Verification items for the finished model (mm, model axes). Face numbers are marked on the shaded views. A direction names the side the tool comes from. Round coordinates to 2 decimals unless told otherwise and drop trailing zeros. Write each loop counter-clockwise with the first axis right and the second up, starting at its lowest first coordinate (ties: lowest second). Pieces come first, ordered by that corner, then holes. Notation, with made-up numbers: M -16.5,53.5 L 13.5,53.5 A12 cw 13.5,74.5 Z; hole C 86,9 d1. An arc over 180 degrees is marked long. Write each question's results on one line, items separated by ' | '.
from build123d import *

# Parameters (mm, degrees)
ESQUISSE2_W             = 44
ESQUISSE2_H             = 44
BOSS_EXTRU_1_DEPTH      = 10
ESQUISSE3_W             = 36
ESQUISSE3_H             = 36
BOSS_EXTRU_2_DEPTH      = 10
ESQUISSE4_W             = 42.5
ESQUISSE4_H             = 42.5
ESQUISSE4_W_2           = 36
ESQUISSE4_H_2           = 36
ENL_V_MAT_EXTRU_1_DEPTH = 5
CONG_1_R                = 3
CONG_2_R                = 2


with BuildPart() as part:
    # Esquisse2 → Boss.-Extru.1 (new body)
    with BuildSketch(Plane.XY):
        with Locations((22, 22)):
            Rectangle(ESQUISSE2_W, ESQUISSE2_H)
    extrude(amount=BOSS_EXTRU_1_DEPTH)

    # Esquisse3 → Boss.-Extru.2 (add)
    with BuildSketch(Plane(origin=(0, 0, 0), x_dir=(-1, 0, 0), z_dir=(0, 0, -1))):
        with Locations((-22, 22)):
            Rectangle(ESQUISSE3_W, ESQUISSE3_H)
    extrude(amount=BOSS_EXTRU_2_DEPTH)

    # Esquisse4 → Enlèv. mat.-Extru.1 (cut)
    with BuildSketch(Plane(origin=(0, 0, 0), x_dir=(-1, 0, 0), z_dir=(0, 0, -1))):
        with Locations((-22.75, 21.25)):
            Rectangle(ESQUISSE4_W, ESQUISSE4_H)
        with Locations((-22, 22)):
            Rectangle(ESQUISSE4_W_2, ESQUISSE4_H_2, mode=Mode.SUBTRACT)
    extrude(amount=-ENL_V_MAT_EXTRU_1_DEPTH, mode=Mode.SUBTRACT)

    # Congé1
    cong_1_edges = [part.edges().sort_by_distance(p)[0] for p in [
        (22, 40, -10),
        (4, 22, -10),
        (22, 4, -10),
        (40, 22, -10),
        (44, 0, 7.5),
        (44, 44, 5),
        (0, 0, 5),
        (0, 44, 5),
        (1.5, 42.5, 2.5),
        (4, 4, -2.5),
        (4, 40, -2.5),
        (40, 4, -2.5),
        (40, 40, -2.5),
    ]]
    fillet(cong_1_edges, radius=CONG_1_R)

    # Congé2
    cong_2_edges = [part.edges().sort_by_distance(p)[0] for p in [
        (44, 22, 10),
        (22, 0, 10),
        (0, 22, 10),
        (22, 44, 10),
        (0.878679656, 43.121320344, 10),
        (0.878679656, 0.878679656, 10),
        (43.121320344, 43.121320344, 10),
        (43.121320344, 0.878679656, 10),
    ]]
    fillet(cong_2_edges, radius=CONG_2_R)


solid = part.part
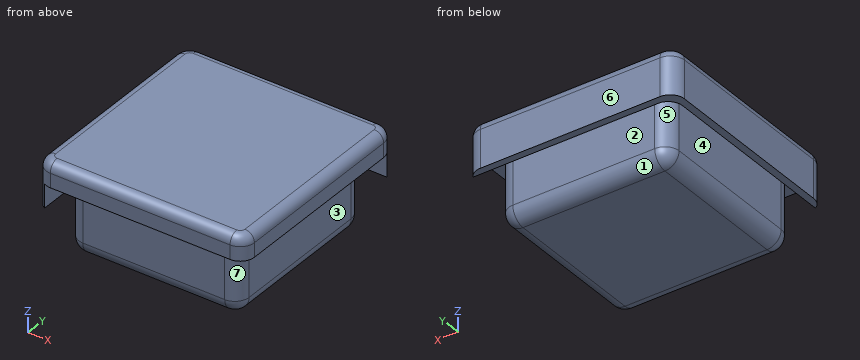
1) Access from +Z, -Z, +X, -X, +Y, -Y to the whole of each face (thin tool, end or side, straight path). Record for the marked faces 1, 2 and 3.
Calculated:
face 1: -Z, +X, -X, +Y | face 2: -Z, +X | face 3: -Z, +X, -Y
2) Depth check by flat-ended pin: P1, Ø3, axis at x = 14, z = 3, coming from the -Y side; P2, Ø5.5, axis at x = 14.5, z = 3, coming from the -Y side; P3, Ø8, axis at y = 20, z = -5, coming from the -X side; P4, Ø3, axis at y = 15.5, z = 1, coming from the +X side. Enter the tip coordinate at first touch or a pass-through.
Calculated:
P1: stops at y = 4 | P2: stops at y = 0 | P3: stops at x = 4 | P4: stops at x = 40
3) Sectioned sample at C-C, the plane z = -5.75. Record the cut outline in (x, y).
Calculated:
outline: M 4,7 A3 ccw 7,4 L 37,4 A3 ccw 40,7 L 40,37 A3 ccw 37,40 L 7,40 A3 ccw 4,37 Z
4) Sectioned sample at A-A, the plane z = 2.75. Record the cut outline in (x, y).
Calculated:
outline: M 0,3 A3 ccw 1.5,0.4 L 1.5,39.5 A3 cw 4.5,42.5 L 43.6,42.5 A3 ccw 41,44 L 3,44 A3 ccw 0,41 Z; M 4,7 A3 ccw 7,4 L 37,4 A3 ccw 40,7 L 40,37 A3 ccw 37,40 L 7,40 A3 ccw 4,37 Z
5) Sectioned sample at B-B, the plane x = 24.5. Record the cut outline in (y, z), and give its area (3 significant figures).
Calculated:
outline: M 0,5 L 4,5 L 4,-7 A3 ccw 7,-10 L 37,-10 A3 ccw 40,-7 L 40,5 L 42.5,5 L 42.5,0 L 44,0 L 44,8 A2 ccw 42,10 L 2,10 A2 ccw 0,8 Z | area: 762 mm²
6) Sectioned sample at D-D, the plane y = 33. Record the cut outline in (x, z), and give its area (3 significant figures).
Calculated:
outline: M 0,0 L 1.5,0 L 1.5,5 L 4,5 L 4,-7 A3 ccw 7,-10 L 37,-10 A3 ccw 40,-7 L 40,5 L 44,5 L 44,8 A2 ccw 42,10 L 2,10 A2 ccw 0,8 Z | area: 762 mm²
7) Draft check along X on the marked faces 4, 5, 6 and 7. Enter one of: pulls with the +X half, pulls with the -X half, needs draft (parallel to the pull), parting line crosses it, or undercut.
Calculated:
face 4: undercut | face 5: undercut | face 6: needs draft | face 7: pulls with the +X half
8) Material ranges on line 1 (X direction, y = 10, z = 2.25); line 2 (Y direction, x = 11, z = 4.5); line 3 (Z direction, x = 2, y = 40.5), recorded low to high. Write a range as [from, to].
Calculated:
line 1: x = [0, 1.5], [4, 40] | line 2: y = [4, 40], [42.5, 44] | line 3: z = [5, 10]
